Build history of the part. All positions in model axes, mm. Round coordinates to 2 decimals unless told otherwise and drop trailing zeros. Order: outer loops, then holes, each group sorted by start corner. A loop starts at its lowest first (then second) coordinate and runs counter-clockwise, first axis right, second up. Notation, with made-up numbers: M 48,47 L 57,47 A28 cw 57,66 Z; hole C 51.5,64.5 d1. An arc over 180 degrees is marked long. One line per item, written item: value. Start each with the question number.
Item 1: Band-saw the part on C-C, the plane x = 34.25. Write the cut outline in (y, z).
Item 2: Probe L1, parallel to X at y = 1.9, z = 52.5; L2, parallel to Y at x = 24, z = 6.5; L3, parallel to X at y = 2.65, z = 18.5. List the from-to ranges inside material, lowest first.
Item 3: Band-saw the part on A-A, the plane z = 50.5. Write the cut outline in (x, y), then the cut area to 3 significant figures.
Item 4: Pin check, flat tips, straight feed: pin 1 (1.1 mm diameter, centred on y = 0.5, z = 61.5, fed in from -X); pin 2 (0.8 mm diameter, centred on y = 1.5, z = 2.5, fed in from -X); pin 3 (0.8 mm diameter, centred on y = 1.5, z = 57.5, fed in from -X). Stop position of each tip, or through.
Item 5: Band-saw the part on B-B, the plane y = 2.45. Write the cut outline in (x, z).
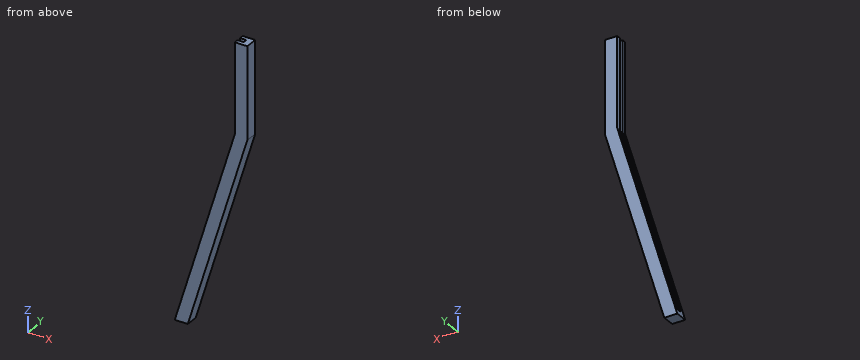
```python
from build123d import *

# Parameters (mm, degrees)
EXTRUDE_1_DEPTH                   = 3
SKETCH_2_R                        = 1.5
SKETCH_2_R_2                      = 0.75
EXTRUDE_2_DEPTH                   = 73
SKETCH_3_W                        = 42
SKETCH_3_H                        = 3.5
SKETCH_3_W_2                      = 3.2
SKETCH_3_H_2                      = 20.2
CUT_EXTRUDE_1_DEPTH               = 83.725086884
CUT_EXTRUDE_2_REACH               = 84.028
CUT_EXTRUDE_2_OFFSET_FROM_SURFACE = 1.5
CUT_EXTRUDE_START                 = -1.5
SKETCH_4_W                        = 44.5
SKETCH_4_H                        = 1
SKETCH_4_3_W                      = 22
SKETCH_4_3_H                      = 1
CUT_EXTRUDE_3_DEPTH               = 37.5
SKETCH_5_W                        = 3
SKETCH_5_H                        = 1
EXTRUDE_3_DEPTH                   = 34.5
SKETCH_6_R                        = 0.35
CUT_EXTRUDE_4_DEPTH               = 80.653562381
SKETCH_7_W                        = 24.036657481
SKETCH_7_H                        = 1
CUT_EXTRUDE_5_DEPTH               = 1.5
SKETCH_8_OUTSIDE_W                = 60.252
SKETCH_8_OUTSIDE_H                = 87.752
CUT_EXTRUDE_6_DEPTH               = 80.653562381


with BuildPart() as part:
    # 草图1 → 凸台-拉伸1 (new body)
    with BuildSketch(Plane(origin=(0, 0, 0), x_dir=(1, 0, 0), z_dir=(0, 1, 0))):
        Polygon((0, 0), (0, -73), (38.8, -73), (38.8, -47.5), (24.5, 0), align=None)
    extrude(amount=EXTRUDE_1_DEPTH)

    # 草图2 → 凸台-拉伸2 (add)
    # profile 1 of 2: a face of its own
    with BuildSketch(Plane(origin=(0, 0, 0), x_dir=(-1, 0, 0), z_dir=(0, 0, -1))):
        with BuildLine():
            Line((0, 3), (0, 0))
            Line((0, 0), (1.7, 0))
            ThreePointArc((1.7, 0), (0.2, 1.5), (1.7, 3))
            Line((1.7, 3), (0, 3))
        make_face()
    # profile 2 of 2: a face of its own
    with BuildSketch(Plane(origin=(0, 0, 0), x_dir=(-1, 0, 0), z_dir=(0, 0, -1))):
        with Locations((1.7, 1.5)):
            Circle(SKETCH_2_R)
        with Locations((1.7, 1.5)):
            Circle(SKETCH_2_R_2, mode=Mode.SUBTRACT)
    extrude(amount=-EXTRUDE_2_DEPTH)

    # 草图3 → 切除-拉伸1 (cut, through all)
    with BuildSketch(Plane(origin=(0, 3, 0), x_dir=(1, 0, 0), z_dir=(0, 1, 0))):
        with Locations((17.8, -71.25)):
            Rectangle(SKETCH_3_W, SKETCH_3_H)
        with Locations((-1.6, -38.1)):
            Rectangle(SKETCH_3_W_2, SKETCH_3_H_2)
        Polygon((1.3, -3), (22.270157068, -3), (35.8, -47.941785964), (35.8, -69.5), (1.3, -69.5), align=None)
    extrude(amount=-CUT_EXTRUDE_1_DEPTH, mode=Mode.SUBTRACT)

    # 切除-拉伸2: up to this face of the body (flat: up to its plane, moved by the offset)
    cut_extrude_2_end = Plane(part.part.faces().sort_by_distance((29.035078534, 1.5, 25.470892982))[0]).offset(-CUT_EXTRUDE_2_OFFSET_FROM_SURFACE)
    # 草图4 → 切除-拉伸2 (cut, up to the picked face)
    with BuildSketch(Plane(origin=(1.3, 0, 0), x_dir=(0, 0, -1), z_dir=(1, 0, 0)).offset(CUT_EXTRUDE_START), mode=Mode.PRIVATE) as cut_extrude_2_sk1:
        with Locations((-25.25, 1.5)):
            Rectangle(SKETCH_4_W, SKETCH_4_H)
    cut_extrude_2_tool1 = split(extrude(cut_extrude_2_sk1.sketch, amount=CUT_EXTRUDE_2_REACH, mode=Mode.PRIVATE), bisect_by=cut_extrude_2_end, keep=Keep.BOTH, mode=Mode.PRIVATE)
    add(cut_extrude_2_tool1.solids().sort_by(Axis((-0.2, 1.5, 25.25), (1, 0, 0)))[0], mode=Mode.SUBTRACT)

    # 草图4<3> → 切除-拉伸3 (cut)
    with BuildSketch(Plane(origin=(1.3, 0, 0), x_dir=(0, 0, -1), z_dir=(1, 0, 0)).offset(CUT_EXTRUDE_START)):
        with Locations((-58.5, 1.5)):
            Rectangle(SKETCH_4_3_W, SKETCH_4_3_H)
    extrude(amount=CUT_EXTRUDE_3_DEPTH, mode=Mode.SUBTRACT)

    # 草图5 → 凸台-拉伸3 (add)
    with BuildSketch(Plane.ZY.offset(-35.8)):
        with Locations((49.441785964, 2.5)):
            Rectangle(SKETCH_5_W, SKETCH_5_H)
    extrude(amount=EXTRUDE_3_DEPTH)

    # 草图6 → 切除-拉伸4 (cut, through all)
    with BuildSketch(Plane(origin=(0, 3, 0), x_dir=(1, 0, 0), z_dir=(0, 1, 0))):
        with Locations(Location((32.8, -49.441785964, 0), (0, 0, 270))):
            Circle(SKETCH_6_R)
        with Locations(Location((24.9, -49.441785964, 0), (0, 0, 270))):
            Circle(SKETCH_6_R)
    extrude(amount=-CUT_EXTRUDE_4_DEPTH, mode=Mode.SUBTRACT)

    # 草图7 → 切除-拉伸5 (cut)
    with BuildSketch(Plane.XY.offset(3)):
        with Locations((11.818328741, 1.5)):
            Rectangle(SKETCH_7_W, SKETCH_7_H)
    extrude(amount=-CUT_EXTRUDE_5_DEPTH, mode=Mode.SUBTRACT)

    # 草图8 outside → 切除-拉伸6 (cut, through all)
    with BuildSketch(Plane(origin=(0, 3, 0), x_dir=(1, 0, 0), z_dir=(0, 1, 0))):
        with Locations((17.8, -34.75)):
            Rectangle(SKETCH_8_OUTSIDE_W, SKETCH_8_OUTSIDE_H)
        Polygon((20.332372981, 3.436695391), (35.8, -47.941785964), (35.8, -72.849501568), (56.307983414, -72.849501568), (56.307983414, 3.436695391), align=None, mode=Mode.SUBTRACT)
    extrude(amount=-CUT_EXTRUDE_6_DEPTH, mode=Mode.SUBTRACT)


solid = part.part
```
Output:
1. outline: M 0,32.39 L 3,32.39 L 3,42.79 L 2,42.79 L 2,37.59 L 1,37.59 L 1,42.79 L 0,42.79 Z
2. L1: x = 37.3 to 38.8
2. L2: y = 0 to 1, 2 to 3
2. L3: x = 26.94 to 30.07
3. outline: M 35.8,0 L 38.8,0 L 38.8,3 L 35.8,3 L 35.8,2 L 37.3,2 L 37.3,1 L 35.8,1 Z
3. area: 7.50 mm²
4. pin 1: stops at x = 35.8
4. pin 2: stops at x = 23.84
4. pin 3: stops at x = 37.3
5. outline: M 21.37,0 L 24.5,0 L 38.8,47.5 L 38.8,69.5 L 35.8,69.5 L 35.8,47.94 Z
